Read the model definition and answer for the solid it produces. Units are mm, in the model's axes. A direction names the side the tool comes from. Coordinates: 2 decimals unless noted, no trailing zeros. Loops run counter-clockwise (first coordinate to the right, second up) from the corner with the lowest first, then second, coordinate; pieces in that order, holes last. Notation, with made-up numbers: M 14,-6.5 L 23,-6.5 A22 cw 23,9.5 Z; hole C -7,-5.5 d4. An arc over 180 degrees is marked long. Use one line per item in the form item = value. Start each with the question number.
1. A tool of negligible diameter and unlimited length cuts with its end or side. For faces 4 (the flat face through (12, -6, 4)), 5 (the cylindrical face through (8.25, 8.21, 8.23)), 6 (the flat face through (12.47, -2.2, 5.42)), from which of +Z, -Z, +X, -X, +Y, -Y can it reach the whole face along a straight path? Write none if from no direction.
2. Find the intervals of material crossed by probe 1 along Y at (x, z) = (0, 7.75); probe 2 along X at (y, z) = (-2.7, 5.5); probe 3 along Y at (x, z) = (-3.25, 4), in increasing order. Write a range as [from, to].
3. The part is cut by section D-D (y = 0). Give the vertices of the cut face in (x, z), plus the area to 3 significant figures.
4. The part is cut by section B-B (y = 13). Give the vertices of the cut face in (x, z).
5. The part is cut by section A-A (x = 0). Give the vertices of the cut face in (y, z), plus the area to 3 significant figures.
6. The part is cut by section C-C (z = 4.5). Give the number of separate pieces and of enclosed holes in the cut face, plus the area to 3 significant figures.
7. For a pull along X with two mould halves and no side action, classify faces 1 (the flat face through (13.4, 6.1, 8)), 2 (the cylindrical face through (8.93, -3.77, 6.28)), 3 (the flat face through (6.689, -11, 6)) as released by +X, released by -X, zero draft, split by the parting line, or undercut.
8. Flat-ended cylindrical pins translate along their axes: pin 1 (3 mm diameter, centred on x = 10.44, z = 5.5, fed in from -Y); pin 2 (4 mm diameter, centred on y = 6, z = 3.5, fed in from +X); pin 3 (1 mm diameter, centred on x = -5.5, z = 8.5, fed in from -Y); pin 4 (1.9 mm diameter, centred on x = 11, z = 7.5, fed in from -Y). Find the tip coordinate at first contact, or state that the pin passes through.
from build123d import *

# Parameters (mm, degrees)
BOSS_EXTRUDE1_DEPTH     = 11
CUT_EXTRUDE1_DEPTH      = 25.021240601
CUT_EXTRUDE1_DEPTH_BACK = 25.021240601
SKETCH3_R               = 1.7
CUT_EXTRUDE2_START      = 5
SKETCH3_3_R             = 3.5
SKETCH3_3_R_2           = 1.7
CUT_EXTRUDE2_DEPTH      = 20.021240772
CUT_EXTRUDE4_START      = -6
SKETCH4_W               = 8.181634888
SKETCH4_H               = 11
CUT_EXTRUDE4_DEPTH      = 19.021240772
FILLET1_SIZE            = 1
FILLET1_SIZE_2          = 3


with BuildPart() as part:
    # Sketch1 → Boss-Extrude1 (new body)
    with BuildSketch(Plane.XY):
        with BuildLine():
            Line((6.007327293, 1.059253884), (14.87059707, 2.622087483))
            ThreePointArc((14.87059707, 2.622087483), (-15.1, 0), (14.87059707, -2.622087483))
            Line((14.87059707, -2.622087483), (6.007327293, -1.059253884))
            ThreePointArc((6.007327293, -1.059253884), (-6.1, 0), (6.007327293, 1.059253884))
        make_face()
    extrude(amount=BOSS_EXTRUDE1_DEPTH)

    # Sketch3 → Cut-Extrude1 (cut, two sides: drawn at the far end of the back side and taken through both)
    with BuildSketch(Plane(origin=(0, 0, 0), x_dir=(1, 0, 0), z_dir=(0, 1, 0)).offset(-CUT_EXTRUDE1_DEPTH_BACK)):
        with Locations(Location((10.438962182, -5.5, 0), (0, 0, 270))):
            Circle(SKETCH3_R)
    extrude(amount=CUT_EXTRUDE1_DEPTH + CUT_EXTRUDE1_DEPTH_BACK, mode=Mode.SUBTRACT)

    # Sketch3<3> → Cut-Extrude2 (cut, through all)
    # profile 1 of 2: a face of its own
    with BuildSketch(Plane(origin=(0, 0, 0), x_dir=(1, 0, 0), z_dir=(0, 1, 0)).offset(CUT_EXTRUDE2_START)):
        with Locations((10.438962182, -5.5)):
            Circle(SKETCH3_3_R)
        with Locations(Location((10.438962182, -5.5, 0), (0, 0, 270))):
            Circle(SKETCH3_3_R_2, mode=Mode.SUBTRACT)
    # profile 2 of 2: a face of its own
    with BuildSketch(Plane(origin=(0, 0, 0), x_dir=(1, 0, 0), z_dir=(0, 1, 0)).offset(CUT_EXTRUDE2_START)):
        with BuildLine():
            Line((6.938962182, 0), (6.938962182, -5.5))
            ThreePointArc((6.938962182, -5.5), (10.438962182, -2), (13.938962182, -5.5))
            ThreePointArc((13.938962182, -5.5), (13.665664376, -6.855873501), (12.888451925, -8))
            Line((12.888451925, -8), (14.87059707, -8))
            Line((14.87059707, -8), (14.87059707, -5.5))
            Line((14.87059707, -5.5), (14.87059707, 0))
            Line((14.87059707, 0), (6.938962182, 0))
        make_face()
    extrude(amount=CUT_EXTRUDE2_DEPTH, mode=Mode.SUBTRACT)

    # Sketch4 → Cut-Extrude4 (cut, through all)
    with BuildSketch(Plane(origin=(0, 0, 0), x_dir=(1, 0, 0), z_dir=(0, 1, 0)).offset(CUT_EXTRUDE4_START)):
        with Locations((10.779779626, -5.5)):
            Rectangle(SKETCH4_W, SKETCH4_H)
    extrude(amount=-CUT_EXTRUDE4_DEPTH, mode=Mode.SUBTRACT)

    # Fillet1
    # an asymmetric fillet: 3, 1 mm, written as the material it adds along each edge
    with BuildSketch(Plane(origin=(6.688962182, -6, 0), x_dir=(1, 0, 0), z_dir=(0, 0, 1))) as fillet1_piece_1:
        with BuildLine():
            Bezier((FILLET1_SIZE, 0), (0, 0), (0, -FILLET1_SIZE_2), weights=[1, 0.707106781, 1])
            Line((0, -FILLET1_SIZE_2), (0, 0))
            Line((0, 0), (FILLET1_SIZE, 0))
        make_face()
    extrude(amount=11)


solid = part.part
Computed values:
q1.face_4 = +Z, -Z, +X, -Y
q1.face_5 = -Z, +Y
q1.face_6 = +Z, -Z, +X
q2.probe_1 = [-15.1, -6.1], [6.1, 15.1]
q2.probe_2 = [-14.86, -5.47], [5.47, 8.74], [12.14, 14.86]
q2.probe_3 = [-14.75, -5.16], [5.16, 14.75]
q3.outline = M -15.1,0 L -6.1,0 L -6.1,11 L -15.1,11 Z
q3.area = 99.0 mm²
q4.outline = M -7.68,0 L 6.94,0 L 6.94,5.5 A3.5 cw 7.68,7.66 L 7.68,11 L -7.68,11 Z
q5.outline = M -15.1,0 L -6.1,0 L -6.1,11 L -15.1,11 Z; M 6.1,0 L 15.1,0 L 15.1,11 L 6.1,11 Z
q5.area = 198 mm²
q6.separate_pieces = 3
q6.enclosed_holes = 0
q6.area = 474 mm²
q7.face_1 = zero draft
q7.face_2 = undercut
q7.face_3 = released by +X
q8.pin_1 = through
q8.pin_2 = 14.56
q8.pin_3 = -14.25
q8.pin_4 = -6
